from build123d import *

# Parameters (mm, degrees)
F0_W     = 80
F0_H     = 100
F0_R     = 7
F1_DEPTH = 5


with BuildPart() as f1:
    # F0 (on Top) → F1 (new body)
    with BuildSketch(Plane.XY):
        Rectangle(F0_W, F0_H)
        with Locations((0, -16.881289)):
            Circle(F0_R, mode=Mode.SUBTRACT)
        with BuildLine():
            Line((-7.573214, -14.20428), (-7.573214, -19.523358))
            Line((-7.573214, -19.523358), (-8.573214, -19.523358))
            Line((-8.573214, -19.523358), (-8.573214, -20.023358))
            Line((-8.573214, -20.023358), (-8.843749, -20.023358))
            ThreePointArc((-8.843749, -20.023358), (-8.900117, -20.021085), (-8.956119, -20.01428))
            Line((-8.956119, -20.01428), (-20.895163, -18.072539))
            ThreePointArc((-20.895163, -18.072539), (-21.195774, -17.902958), (-21.314899, -17.579023))
            Line((-21.314899, -17.579023), (-21.314899, -17.160009))
            Line((-21.314899, -17.160009), (-21.314899, -15.299222))
            ThreePointArc((-21.314899, -15.299222), (-21.24047, -14.857391), (-21.0254, -14.464328))
            Line((-21.0254, -14.464328), (-21.0254, -14.01055))
            Line((-21.0254, -14.01055), (-21.0254, -12.913586))
            Line((-21.0254, -12.913586), (-21.0254, -9.813586))
            Line((-21.0254, -9.813586), (-21.0254, -9.767418))
            Line((-21.0254, -9.767418), (-21.197006, -9.2368))
            Line((-21.197006, -9.2368), (-20.653205, 13.45957))
            Line((-20.653205, 13.45957), (-20.653205, 13.747156))
            ThreePointArc((-20.653205, 13.747156), (-20.61125, 13.910455), (-20.495776, 14.033308))
            ThreePointArc((-20.495776, 14.033308), (-19.935874, 14.323579), (-19.334331, 14.513035))
            Line((-19.334331, 14.513035), (-18.223464, 14.782686))
            ThreePointArc((-18.223464, 14.782686), (-18.134694, 14.76198), (-18.098606, 14.678275))
            Line((-18.098606, 14.678275), (-18.638507, -7.855344))
            ThreePointArc((-18.638507, -7.855344), (-18.764323, -7.869872), (-18.888049, -7.896943))
            ThreePointArc((-18.888049, -7.896943), (-19.459477, -8.105502), (-19.987784, -8.407029))
            ThreePointArc((-19.987784, -8.407029), (-19.458243, -8.167158), (-18.888049, -8.053886))
            ThreePointArc((-18.888049, -8.053886), (-18.201931, -8.25824), (-17.834234, -8.872502))
            Line((-17.834234, -8.872502), (-16.653947, -12.861871))
            ThreePointArc((-16.653947, -12.861871), (-16.664462, -13.422165), (-16.995338, -13.874449))
            ThreePointArc((-16.995338, -13.874449), (-17.045524, -13.901224), (-17.101217, -13.912787))
            Line((-17.101217, -13.912787), (-16.810631, -13.894739))
            Line((-16.810631, -13.894739), (-16.340575, -13.894739))
            ThreePointArc((-16.340575, -13.894739), (-16.237071, -13.701517), (-16.164339, -13.494739))
            Line((-16.164339, -13.494739), (-15.217034, -13.494739))
            Line((-15.217034, -13.494739), (-14.968154, -13.494739))
            Line((-14.968154, -13.494739), (-8.566029, -13.494739))
            Line((-8.566029, -13.494739), (-8.566029, -13.894739))
            ThreePointArc((-8.566029, -13.894739), (-7.549092, -10.652508), (-5.067064, -8.331785))
            Line((-5.067064, -8.331785), (0.704507, -6.687392))
            ThreePointArc((0.704507, -6.687392), (1.902164, -6.547103), (3.082686, -6.792931))
            ThreePointArc((3.082686, -6.792931), (6.192475, -8.520067), (8.700256, -11.042926))
            Line((8.700256, -11.042926), (26.258714, -11.042926))
            Line((26.258714, -11.042926), (26.258714, -14.213515))
            Line((26.258714, -14.213515), (26.258714, -18.120132))
            Line((26.258714, -18.120132), (25.466068, -19.523358))
            Line((25.466068, -19.523358), (9.943894, -19.209119))
            Line((9.943894, -19.209119), (9.943894, -19.523358))
            Line((9.943894, -19.523358), (8.943894, -19.523358))
            Line((8.943894, -19.523358), (8.943894, -13.664436))
            ThreePointArc((8.943894, -13.664436), (8.835951, -13.194662), (8.636425, -12.755881))
            ThreePointArc((8.636425, -12.755881), (6.1104, -9.735893), (2.724563, -7.726606))
            ThreePointArc((2.724563, -7.726606), (1.857829, -7.54612), (0.978515, -7.649119))
            Line((0.978515, -7.649119), (-4.684119, -9.262475))
            ThreePointArc((-4.684119, -9.262475), (-6.797948, -11.342099), (-7.573214, -14.20428))
        make_face(mode=Mode.SUBTRACT)
    extrude(amount=-F1_DEPTH)


solid = f1.part
CAD build for the part. Positions are in the model's coordinates, mm. A direction names the side the tool comes from. Coordinates: 2 decimals unless noted, no trailing zeros. Order: outer loops, then holes, each group sorted by start corner. A loop starts at its lowest first (then second) coordinate and runs counter-clockwise, first axis right, second up.
Item 1: Pin check, flat tip, straight feed: pin 1 Ø11 at (x, y) = (0, -16.88) entering from -Z. Stop position of the tip, or through.
Check sheet entries:
pin 1: passes through
Item 2: Two-plate mould, pull along Y, no slides. Class faces 3 (the face through (40, -1, -2)), 4 (the face through (-7.573, -17, -2)), 5 (the face through (-1, -50, -2)): +Y half, -Y half, draft (parallel to the pull), parting line (faces both ways), or undercut.
Check sheet entries:
face 3: draft
face 4: undercut
face 5: -Y half
Item 3: 3-axis set-ups, long thin cutter, end or side, ignore diameter. For faces 1 (the face through (-1.813, -8.445, -2.465)), 2 (the face through (-1, 50, -2)): which of +Z, -Z, +X, -X, +Y, -Y reach the whole face in a straight line?
Check sheet entries:
face 1: +Z, -Z
face 2: +Z, -Z, +X, -X, +Y
Item 4: Band-saw the part on B-B on y = 11. List the corners of the cut face in (x, z), plus the area to 3 significant figures.
Check sheet entries:
outline: (-40, -5) - (-20.71, -5) - (-20.71, 0) - (-40, 0) - close; (-18.19, -5) - (40, -5) - (40, 0) - (-18.19, 0) - close
area: 387 mm2
Item 5: Drill centre lines: L1, parallel to Y at x = 0, z = -2.9; L2, parallel to Y at x = 3, z = -0.9; L3, parallel to X at y = -14, z = -1.25. Where is each one in solid material? Low to high.
Check sheet entries:
L1: y = -50 to -23.88, -9.88 to -7.93, -6.89 to 50
L2: y = -50 to -23.21, -10.56 to -7.84, -6.76 to 50
L3: x = -40 to -21.03, -7.57 to -6.38, 6.38 to 8.94, 26.26 to 40
Item 6: Band-saw the part on A-A on x = 15. List the corners of the cut face in (y, z), plus the area to 3 significant figures.
Check sheet entries:
outline: (-50, -5) - (-19.31, -5) - (-19.31, 0) - (-50, 0) - close; (-11.04, -5) - (50, -5) - (50, 0) - (-11.04, 0) - close
area: 459 mm2
Item 7: Band-saw the part on C-C on z = -1.55. Give the number of separate pieces and of enclosed holes in the cut face, plus the area to 3 significant figures.
Check sheet entries:
separate pieces: 1
enclosed holes: 2
area: 7,530 mm2
